Can you work these out from the model? Positions are in its coordinate system, mm. A direction names the side the tool comes from. Round coordinates to 2 decimals unless told otherwise and drop trailing zeros. Write each loop counter-clockwise with the first axis right and the second up, starting at its lowest first coordinate (ties: lowest second). Pieces come first, ordered by that corner, then holes. Notation, with made-up numbers: M 65.25,34.5 L 113.25,34.5 A25 cw 113.25,65.5 Z; hole C -15.75,63 d8. An arc over 180 degrees is marked long. Answer as a JSON object with one key per item and string values. Group by question number.
1) Please list where these lines run through material, in increasing order: L1, parallel to Y at x = -2.5, z = 1.65; L2, parallel to X at y = 2.5, z = 2.25; L3, parallel to Y at x = 12.5, z = 1.6. Write a range as [from, to].
2) I'm going to push flat-ended pins straight in: pin 1 Ø1 at (y, z) = (-44, 1) entering from -X; pin 2 Ø6 at (x, y) = (-0.7, -30.48) entering from +Z; pin 3 Ø1.6 at (x, z) = (-19, 2) entering from -Y; pin 4 Ø1.5 at (x, z) = (10.5, 2) entering from -Y. Where does each tip first touch, or does it pass through?
3) Suppose I cut it at C-C, the plane y = -30.48. Write out the boundary of the cut face in (x, z) (3 decimals).
4) If we mould it in two halves opening along Y, with no side actions, what happens to faces 1 (the flat face through (-3.175, -43, 2)), 2 (the flat face through (-19, 13.723, 2)), 3 (the flat face through (-14.87, -34.61, 1.57)), 4 (the flat face through (-23.626, 1.114, 1.565))? For each: +Y half, -Y half, draft (parallel to the pull), parting line (faces both ways), or undercut.
5) Suppose I cut it at B-B, the plane x = 0. Write out the boundary of the cut face in (y, z) (3 decimals).
6) On a 3-axis mill with a long thin cutter (end or side, diameter ignored), from which of +Z, -Z, +X, -X, +Y, -Y can I reach the whole of each face in a straight line? I mean faces 5 (the flat face through (3.175, -43, 2)), 6 (the flat face through (0, -23, 3.175)), 7 (the cylindrical face through (-0.282, 22.223, 1.565)). Say none if no direction works.
7) Suppose I cut it at A-A, the plane z = 2.65. Write out the boundary of the cut face in (x, y) (3 decimals).
8) Suppose I cut it at D-D, the plane x = 12.5. Write out the boundary of the cut face in (y, z) (3 decimals).
from build123d import *

# Parameters (mm, degrees)
F0_R     = 3.233186
F1_DEPTH = 3.175


with BuildPart() as f1:
    # F0 (on Top) → F1 (new body)
    with BuildSketch(Plane.XY):
        with BuildLine():
            Line((24.698584, -24.693283), (24.761808, -24.629424))
            ThreePointArc((24.761808, -24.629424), (0.030307, 34.924987), (-24.804516, -24.586411))
            Line((-24.804516, -24.586411), (-4.650402, -44.919312))
            ThreePointArc((-4.650402, -44.919312), (-3.952362, -45.530209), (-3.175, -46.036336))
            Line((-3.175, -46.036336), (-3.175, -40.3098))
            ThreePointArc((-3.175, -40.3098), (0, -37.1348), (3.175, -40.3098))
            Line((3.175, -40.3098), (3.175, -46.036336))
            ThreePointArc((3.175, -46.036336), (3.952362, -45.530209), (4.650402, -44.919312))
            Line((4.650402, -44.919312), (24.698584, -24.693283))
        make_face()
        with Locations((-0.703903, -30.48)):
            Circle(F0_R, mode=Mode.SUBTRACT)
        with BuildLine():
            ThreePointArc((22.180412, -1.4071), (0.032937, -22.224976), (-22.176144, -1.472834))
            Line((-22.176144, -1.472834), (-25.118009, 3.774338))
            ThreePointArc((-25.118009, 3.774338), (-23.772102, 8.946907), (-21.373594, 13.723318))
            Line((-21.373594, 13.723318), (-17.482024, 13.723318))
            ThreePointArc((-17.482024, 13.723318), (0, 22.225), (17.482024, 13.723318))
            Line((17.482024, 13.723318), (21.373594, 13.723318))
            ThreePointArc((21.373594, 13.723318), (23.772102, 8.946907), (25.118009, 3.774338))
            Line((25.118009, 3.774338), (22.180412, -1.4071))
        make_face(mode=Mode.SUBTRACT)
    extrude(amount=F1_DEPTH)


solid = f1.part
Results:
{
 "1": {"L1": "[-38.35, -33.17], [-27.79, -22.08], [22.08, 34.84]", "L2": "[-34.84, -24.4], [24.4, 34.84]", "L3": "[-37, -18.38], [18.38, 32.61]"},
 "2": {"pin 1": "x = -6.06", "pin 2": "through", "pin 3": "y = -31.25", "pin 4": "y = -39.77"},
 "3": {"outline": "M -18.963,0 L -3.937,0 L -3.937,3.175 L -18.963,3.175 Z; M 2.529,0 L 18.963,0 L 18.963,3.175 L 2.529,3.175 Z"},
 "4": {"face 1": "draft", "face 2": "undercut", "face 3": "-Y half", "face 4": "undercut"},
 "5": {"outline": "M -37.135,0 L -33.636,0 L -33.636,3.175 L -37.135,3.175 Z; M -27.324,0 L -22.225,0 L -22.225,3.175 L -27.324,3.175 Z; M 22.225,0 L 34.925,0 L 34.925,3.175 L 22.225,3.175 Z"},
 "6": {"face 5": "+Z, -Z, -Y", "face 6": "+Z, +X, -X, +Y, -Y", "face 7": "+Z, -Z"},
 "7": {"outline": "M -24.805,-24.586 L -4.65,-44.919 A6.548 ccw -3.175,-46.036 L -3.175,-40.31 A3.175 cw 3.175,-40.31 L 3.175,-46.036 A6.548 ccw 4.65,-44.919 L 24.699,-24.693 L 24.762,-24.629 A34.925 ccw long Z; hole M -25.118,3.774 L -22.176,-1.473 A22.225 ccw 22.18,-1.407 L 25.118,3.774 A25.4 ccw 21.374,13.723 L 17.482,13.723 A22.225 ccw -17.482,13.723 L -21.374,13.723 A25.4 ccw Z; hole C -0.704,-30.48 d6.466"},
 "8": {"outline": "M -37,0 L -18.377,0 L -18.377,3.175 L -37,3.175 Z; M 18.377,0 L 32.611,0 L 32.611,3.175 L 18.377,3.175 Z"}
}
